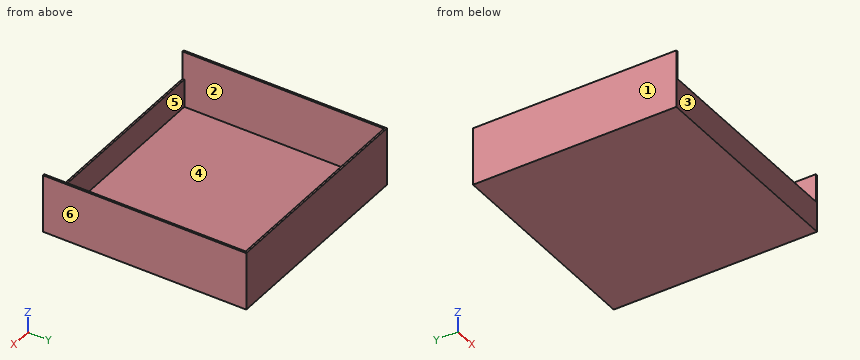
Autodesk Inventor part; units mm, degrees
ref_plane "YZ Plane" through (0, 0, 0) normal (1, 0, 0) x (0, 1, 0)
ref_plane "XZ Plane" through (0, 0, 0) normal (0, 1, 0) x (-1, 0, 0)
ref_plane "XY Plane" through (0, 0, 0) normal (0, 0, 1) x (1, 0, 0)
sketch "Sketch1" plane through (0, 0, 0) normal (0, 0, 1) x (1, 0, 0)
  line L0 (0, 0) -> (187.325, 0)
  line L1 (187.325, 0) -> (187.325, 177.8)
  line L2 (187.325, 177.8) -> (0, 177.8)
  line L3 (0, 177.8) -> (0, 0)
  dimension "d0" = 177.8
  dimension "d1" = 187.325
extrude "Extrusion1" add sketch "Sketch1" along normal blind 50.8
shell "Shell1" thickness 1.5875 removed faces 1 at (124.8833, 59.2667, 50.8)
sketch "Sketch2" plane through (0, 0, 0) normal (0, -1, 0) x (1, 0, 0)
  line L0 (185.7375, 1.5875) -> (185.7375, 50.8)
  line L1 (1.5875, 50.8) -> (185.7375, 50.8)
  line L2 (185.7375, 50.8) -> (185.7375, 26.1937)
  line L3 (185.7375, 26.1937) -> (1.5875, 26.1937)
  line L4 (1.5875, 26.1937) -> (1.5875, 50.8)
  line L5 (1.5875, 1.5875) -> (1.5875, 50.8)
  line L6 (0, 50.8) -> (187.325, 50.8)
  point P0 (0, 0)
  point P1 (1.5875, 26.1937)
  point P2 (93.6625, 50.8)
extrude "Extrusion2" cut sketch "Sketch2" against normal up to surface (1.5875 mm away)
properties part number "BatteryHolder-ver1-1111-2019" material "Aluminum 6061"
Source: CAD feature listing. Evaluate the final solid. Frame: model axes, mm. Face numbers are marked on the shaded views. A direction names the side the tool comes from. Give positions to 0.01 mm unless a question says otherwise; leave off trailing zeros. Write each loop counter-clockwise with the first axis right and the second up, starting at its lowest first coordinate (ties: lowest second). Pieces come first, ordered by that corner, then holes. Notation, with made-up numbers: M -31,5.5 L -6,5.5 A17 ccw -6,9.5 Z; hole C -6.5,18.25 d11. An arc over 180 degrees is marked long. Return JSON: item names as keys, results as strings. Group by question number.
1) Cut plane A-A, the plane x = 145. Output: boundary loops of the cut face in (y, z), then the cut area to 3 significant figures.
2) Set-up query: the marked faces 5 and 6. Return all of +Z, -Z, +X, -X, +Y, -Y with unobstructed straight access to the full face (end or side cutting, diameter ignored); none if empty.
3) Cut plane B-B, the plane z = 18. Output: boundary loops of the cut face in (x, y) (1 decimal).
4) Cut plane C-C, the plane z = 33. Output: boundary loops of the cut face in (x, y) (1 decimal), then the cut area to 3 significant figures.
5) Draft query along X for the marked faces 1, 2, 3 and 4. Return one class per face: released by +X, released by -X, zero draft, split by the parting line, or undercut.
6) First-contact query: pin 1 Ø10 at (x, y) = (42.5, 70) entering from +Z; pin 2 Ø0.8 at (x, y) = (124.5, 1) entering from +Z. Flat tips, straight axial feed; report the tip coordinate or a pass-through.
7) Ray query, L1, parallel to X at y = 16, z = 20 (1 decimal); L2, parallel to Y at x = 25, z = 22; L3, parallel to Z at x = 175, y = 66. Return the intervals inside material, ascending.
Data:
{
 "1": {"outline": "M 0,0 L 177.8,0 L 177.8,50.8 L 176.21,50.8 L 176.21,1.59 L 1.59,1.59 L 1.59,26.19 L 0,26.19 Z", "area": "399 mm²"},
 "2": {"face 5": "+Z", "face 6": "+Z, -Z, +X, +Y, -Y"},
 "3": {"outline": "M 0,0 L 187.3,0 L 187.3,177.8 L 0,177.8 Z; hole M 1.6,1.6 L 185.7,1.6 L 185.7,176.2 L 1.6,176.2 Z"},
 "4": {"outline": "M 0,0 L 1.6,0 L 1.6,176.2 L 185.7,176.2 L 185.7,0 L 187.3,0 L 187.3,177.8 L 0,177.8 Z", "area": "857 mm²"},
 "5": {"face 1": "released by -X", "face 2": "undercut", "face 3": "zero draft", "face 4": "undercut"},
 "6": {"pin 1": "stops at z = 1.59", "pin 2": "stops at z = 26.19"},
 "7": {"L1": "x = 0 to 1.6, 185.7 to 187.3", "L2": "y = 0 to 1.59, 176.21 to 177.8", "L3": "z = 0 to 1.59"}
}
